Read the model definition and answer for the solid it produces. Units are mm, in the model's axes. Face numbers are marked on the shaded views. Coordinates: 2 decimals unless noted, no trailing zeros. Write each loop counter-clockwise with the first axis right and the second up, starting at its lowest first coordinate (ties: lowest second). Pieces come first, ordered by that corner, then holes. Notation, with made-up numbers: (-9.75, -8.75) -> (12.25, -8.75) arc R26 ccw to (12.25, 5.25) -> close; hole circle Ø1 at (28.25, -21.5). An arc over 180 degrees is marked (long way). One line per item, written item: value. Start each with the question number.
from build123d import *

# Parameters (mm, degrees)
F0_W      = 253
F0_H      = 277
F1_DEPTH  = 178
F2_W      = 248
F2_H      = 173
F2_R      = 37.5
F3_DEPTH  = 5
F5_DEPTH  = 15
F6_DEPTH  = 10
F7_R      = 18.5
F8_DEPTH  = 257
F9_R      = 2.2
F10_DEPTH = 5


with BuildPart() as f1:
    # F0 (on Top) → F1 (new body)
    with BuildSketch(Plane.XY):
        Rectangle(F0_W, F0_H)
    extrude(amount=F1_DEPTH)

    # F2 (on face) → F3 (cut)
    with BuildSketch(Plane.XZ.offset(138.5)):
        with Locations((0, 89)):
            Rectangle(F2_W, F2_H)
        with Locations((46, 88.5)):
            Circle(F2_R, mode=Mode.SUBTRACT)
    extrude(amount=-F3_DEPTH, mode=Mode.SUBTRACT)

    # F4 (on face) → F5 (join)
    with BuildSketch(Plane.XZ.offset(138.5)):
        Polygon((-126.5, 178), (-126.5, 88.5), (-124, 88.5), (-124, 175.5), (124, 175.5), (124, 88.5), (126.5, 88.5), (126.5, 178), align=None)
    extrude(amount=F5_DEPTH)

    # F6 (cut): a face of the model
    f6_faces = [f1.faces().sort_by_distance(p)[0] for p in [
        (46, -138.5, 88.5),
    ]]
    extrude(f6_faces, amount=-F6_DEPTH, mode=Mode.SUBTRACT)

    # F7 (on face) → F8 (cut)
    with BuildSketch(Plane.XZ.offset(128.5)):
        with Locations((46, 88.5)):
            Circle(F7_R)
    extrude(amount=-F8_DEPTH, mode=Mode.SUBTRACT)

    # F9 (on face) → F10 (cut)
    with BuildSketch(Plane(origin=(0, 0, 0), x_dir=(1, 0, 0), z_dir=(0, 0, -1))):
        with Locations((-96, 109.0106)):
            Circle(F9_R)
        with Locations((95.9986, 109.0106)):
            Circle(F9_R)
        with Locations((-96, -108.9976)):
            Circle(F9_R)
        with Locations((95.9986, -108.9976)):
            Circle(F9_R)
    extrude(amount=-F10_DEPTH, mode=Mode.SUBTRACT)


solid = f1.part
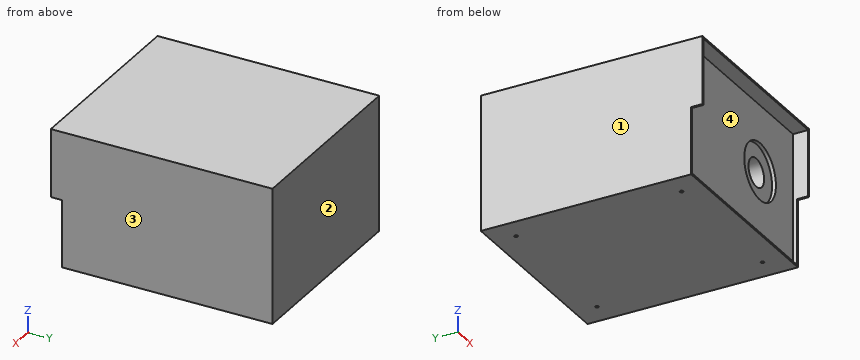
1. For a pull along X with two mould halves and no side action, classify the marked faces 1, 2, 3 and 4 as +X half, -X half, draft (parallel to the pull), parting line (faces both ways), or undercut.
2. A cutting plane is placed at D-D on x = 46. Give the vertices of the cut face in (y, z), then the cut area to 3 significant figures.
3. A cutting plane is placed at B-B on y = -61. Give the vertices of the cut face in (x, z).
4. Given pin 1 (1.2 mm diameter, centred on x = 125.5, y = -144.5, fed in from -Z); pin 2 (10 mm diameter, centred on x = -10, z = 32.5, fed in from -Y); pin 3 (2 mm diameter, centred on x = -96.5, y = -109, fed in from -Z); pin 4 (7 mm diameter, centred on x = -96, y = -109.01, fed in from -Z), each flat-ended and moving along its own axis, determine where each tip first touches the part or whether it passes through.
5. A cutting plane is placed at C-C on z = 162. Give the vertices of the cut face in (x, y), then the cut area to 3 significant figures.
6. Find the intervals of material crossed by probe 1 along Y at (x, z) = (-96, 2); probe 2 along Y at (x, z) = (-96, 2.8); probe 3 along Y at (x, z) = (-3, 133.5), in increasing order. Write a range as from..to.
7. A cutting plane is placed at A-A on x = -24. Give the vertices of the cut face in (y, z).
Derived:
1. face 1: -X half
1. face 2: draft
1. face 3: +X half
1. face 4: undercut
2. outline: (-153.5, 175.5) -> (-133.5, 175.5) -> (-133.5, 126) -> (-128.5, 126) -> (-128.5, 107) -> (128.5, 107) -> (128.5, 70) -> (-128.5, 70) -> (-128.5, 51) -> (-133.5, 51) -> (-133.5, 2.5) -> (-138.5, 2.5) -> (-138.5, 0) -> (138.5, 0) -> (138.5, 178) -> (-153.5, 178) -> close
2. area: 38,600 mm2
3. outline: (-126.5, 0) -> (126.5, 0) -> (126.5, 178) -> (-126.5, 178) -> close; hole circle Ø37 at (46, 88.5)
4. pin 1: stops at z = 88.5
4. pin 2: stops at y = -133.5
4. pin 3: stops at z = 5
4. pin 4: stops at z = 0
5. outline: (-126.5, -153.5) -> (-124, -153.5) -> (-124, -133.5) -> (124, -133.5) -> (124, -153.5) -> (126.5, -153.5) -> (126.5, 138.5) -> (-126.5, 138.5) -> close
5. area: 68,900 mm2
6. probe 1: y = -138.5..-111.21, -106.81..106.8, 111.2..138.5
6. probe 2: y = -133.5..-111.21, -106.81..106.8, 111.2..138.5
6. probe 3: y = -133.5..138.5
7. outline: (-153.5, 175.5) -> (-133.5, 175.5) -> (-133.5, 2.5) -> (-138.5, 2.5) -> (-138.5, 0) -> (138.5, 0) -> (138.5, 178) -> (-153.5, 178) -> close
